```python
from build123d import *

# Parameters (mm, degrees)
SKETCH1_W           = 319.0875
SKETCH1_H           = 88.9
BOSS_EXTRUDE1_DEPTH = 38.1
SKETCH2_W           = 88.9
SKETCH2_H           = 50.8
BOSS_EXTRUDE2_DEPTH = 38.1


with BuildPart() as part:
    # Sketch1 → Boss-Extrude1 (new body)
    with BuildSketch(Plane(origin=(0, 0, 0), x_dir=(1, 0, 0), z_dir=(0, 1, 0))):
        with Locations((159.54375, 44.45)):
            Rectangle(SKETCH1_W, SKETCH1_H)
    extrude(amount=BOSS_EXTRUDE1_DEPTH)

    # Sketch2 → Boss-Extrude2 (add, through all)
    with BuildSketch(Plane.XZ):
        with Locations((363.5375, -25.4)):
            Rectangle(SKETCH2_W, SKETCH2_H)
    extrude(amount=-BOSS_EXTRUDE2_DEPTH)


solid = part.part
```
Design review of the part built by this model. Coordinates are the model's own, in mm. A direction names the side the tool comes from. Round coordinates to 2 decimals unless told otherwise and drop trailing zeros. Write each loop counter-clockwise with the first axis right and the second up, starting at its lowest first coordinate (ties: lowest second). Pieces come first, ordered by that corner, then holes. Notation, with made-up numbers: (82, 86) -> (104, 86) arc R16 cw to (104, 94) -> close; hole circle Ø1 at (43.5, 59). An arc over 180 degrees is marked (long way). Write item = value, one per line. Start each with the question number.
1) Clearance check with flat-ended pins moving along their axes: pin 1 (19 mm diameter, centred on x = 355, y = 10.5, fed in from -Z); pin 2 (3 mm diameter, centred on y = 5, z = -74.5, fed in from +X). State where each tip first meets the part, or that it passes through.
2) Tool access review of faces 1 (the face through (0, 19, -44)), 2 (the face through (319.088, 19, -70)): name each direction out of +Z, -Z, +X, -X, +Y, -Y from which nothing blocks a thin tool from reaching the whole face with its end or side.
3) Take a section at A-A, the plane y = 34.5. State the section outline as (x, z) points, plus the area to 3 significant figures.
4) Take a section at B-B, the plane z = -61.5. State the section outline as (x, y) points, plus the area to 3 significant figures.
5) Take a section at C-C, the plane x = 352. State the section outline as (y, z) points, plus the area to 3 significant figures.
6) Wall thickness on probe 1 along X at (y, z) = (22.5, -75); probe 2 along Z at (x, y) = (321, 10.5): over which ranges is each line inside the solid? List them lowest first. Write a range as from..to.
Results list:
q1.pin_1 = -50.8
q1.pin_2 = 319.09
q2.face_1 = +Z, -Z, -X, +Y, -Y
q2.face_2 = -Z, +X, +Y, -Y
q3.outline = (0, -88.9) -> (319.09, -88.9) -> (319.09, -50.8) -> (407.99, -50.8) -> (407.99, 0) -> (0, 0) -> close
q3.area = 32,900 mm²
q4.outline = (0, 0) -> (319.09, 0) -> (319.09, 38.1) -> (0, 38.1) -> close
q4.area = 12,200 mm²
q5.outline = (0, -50.8) -> (38.1, -50.8) -> (38.1, 0) -> (0, 0) -> close
q5.area = 1,940 mm²
q6.probe_1 = 0..319.09
q6.probe_2 = -50.8..0
